Design review of the part built by this model. Coordinates are the model's own, in mm. Face numbers are marked on the shaded views. A direction names the side the tool comes from. Round coordinates to 2 decimals unless told otherwise and drop trailing zeros. Loops run counter-clockwise (first coordinate to the right, second up) from the corner with the lowest first, then second, coordinate; pieces in that order, holes last. Notation, with made-up numbers: (69.25, -28.5) - (115.25, -28.5) arc R8 ccw to (115.25, -24.5) - close; hole circle Ø2 at (-0.75, 79.5). An arc over 180 degrees is marked (long way). Return JSON: item names as keys, results as strings. Group by question number.
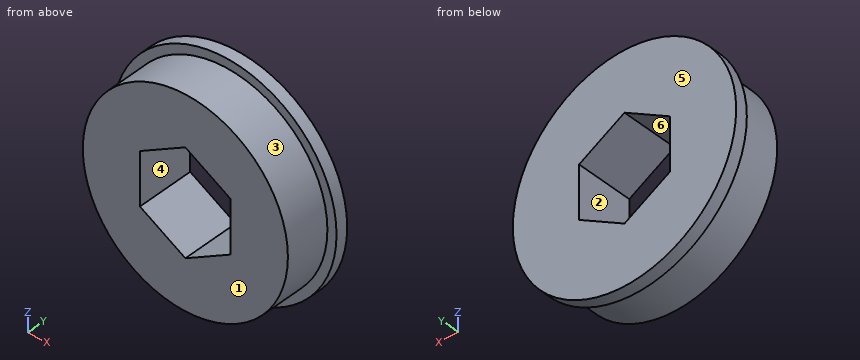
Autodesk Inventor part; units mm, degrees
ref_plane "YZ Plane" through (0, 0, 0) normal (1, 0, 0) x (0, 1, 0)
ref_plane "XZ Plane" through (0, 0, 0) normal (0, 1, 0) x (-1, 0, 0)
ref_plane "XY Plane" through (0, 0, 0) normal (0, 0, 1) x (1, 0, 0)
sketch "Sketch1" plane through (0, 0, 0) normal (0, 1, 0) x (-1, 0, 0)
  circle A0 centre (0, 0) radius 14.31
  line L0 (0, 0) -> (6.335, 0)
  line L1 (6.335, -3.6575) -> (0, -7.315)
  line L2 (0, -7.315) -> (-6.335, -3.6575)
  line L3 (-6.335, -3.6575) -> (-6.335, 3.6575)
  line L4 (-6.335, 3.6575) -> (0, 7.315)
  line L5 (0, 7.315) -> (6.335, 3.6575)
  line L6 (6.335, 3.6575) -> (6.335, -3.6575)
  dimension "d0" = 28.62
  dimension "d1" = 6.335
extrude "Extrusion1" add sketch "Sketch1" along normal blind 8
sketch "Sketch2" plane through (0, 8, 0) normal (0, 1, 0) x (1, 0, 0)
  circle A0 centre (0, 0) radius 15.585
  line L0 (-6.335, -3.6575) -> (-6.335, 3.6575)
  line L1 (-6.335, 3.6575) -> (0, 7.315)
  line L2 (0, 7.315) -> (6.335, 3.6575)
  line L3 (6.335, 3.6575) -> (6.335, -3.6575)
  line L4 (6.335, -3.6575) -> (0, -7.315)
  line L5 (0, -7.315) -> (-6.335, -3.6575)
  line L6 (-6.335, -3.6575) -> (-6.335, 3.6575)
  point P0 (-6.335, 0)
  dimension "d4" = 31.17
extrude "Extrusion2" add sketch "Sketch2" against normal blind 1.7
properties part number "Bearing"
Q1. For line 1 (X direction, y = 2, z = 3) (3 decimals); line 2 (Y direction, x = -5, z = 14.5); line 3 (X direction, y = 3.75, z = -1) (3 decimals), list the stretches that pass through material, from the lowest coordinate up.
Q2. Draft analysis for pull direction X (two halves, no side actions). For the marked faces 1, 2, 3 and 4, state which applies: pulls with the +X half, pulls with the -X half, needs draft (parallel to the pull), parting line crosses it, or undercut.
Q3. Add section C-C, the plane x = -3.5. State the section outline as (y, z) points.
Q4. Add section A-A, the plane z = 0. State the section outline as (x, y) points (3 decimals), plus the area to 3 significant figures.
Q5. Insertion check: pin 1 Ø2 at (y, z) = (4.5, 1) entering from +X; pin 2 Ø4 at (x, z) = (7.5, 8) entering from -Y; pin 3 Ø2 at (y, z) = (4.5, -0.5) entering from -X. Each pin has a flat end and moves straight along its axis. Give the tip position at first contact, or say it passes through.
Q6. Add section D-D, the plane z = 9.5. State the section outline as (x, y) points, plus the area to 3 significant figures.
Q7. Tool access review of the marked faces 5 and 6: name each direction out of +Z, -Z, +X, -X, +Y, -Y from which nothing blocks a thin tool from reaching the whole face with its end or side.
Q8. Add section B-B, the plane y = 7.5. State the section outline as (x, z) points (1 decimal).
Evaluation:
{
 "1": {"line 1": "-13.992 to -6.335, 6.335 to 13.992", "line 2": "6.3 to 8", "line 3": "-14.275 to -6.335, 6.335 to 14.275"},
 "2": {"face 1": "needs draft", "face 2": "undercut", "face 3": "parting line crosses it", "face 4": "undercut"},
 "3": {"outline": "(0, -13.88) - (6.3, -13.88) - (6.3, -15.19) - (8, -15.19) - (8, -5.29) - (0, -5.29) - close; (0, 5.29) - (8, 5.29) - (8, 15.19) - (6.3, 15.19) - (6.3, 13.88) - (0, 13.88) - close"},
 "4": {"outline": "(-15.585, 6.3) - (-14.31, 6.3) - (-14.31, 0) - (-6.335, 0) - (-6.335, 8) - (-15.585, 8) - close; (6.335, 0) - (14.31, 0) - (14.31, 6.3) - (15.585, 6.3) - (15.585, 8) - (6.335, 8) - close", "area": "132 mm²"},
 "5": {"pin 1": "x = 14.31", "pin 2": "y = 0", "pin 3": "x = -14.31"},
 "6": {"outline": "(-12.35, 6.3) - (-10.7, 6.3) - (-10.7, 0) - (10.7, 0) - (10.7, 6.3) - (12.35, 6.3) - (12.35, 8) - (-12.35, 8) - close", "area": "177 mm²"},
 "7": {"face 5": "+Z, -Z, +X, -X, +Y", "face 6": "+Y, -Y"},
 "8": {"outline": "circle Ø31.2 at (0, 0); hole (-6.3, -3.7) - (0, -7.3) - (6.3, -3.7) - (6.3, 3.7) - (0, 7.3) - (-6.3, 3.7) - close"}
}
